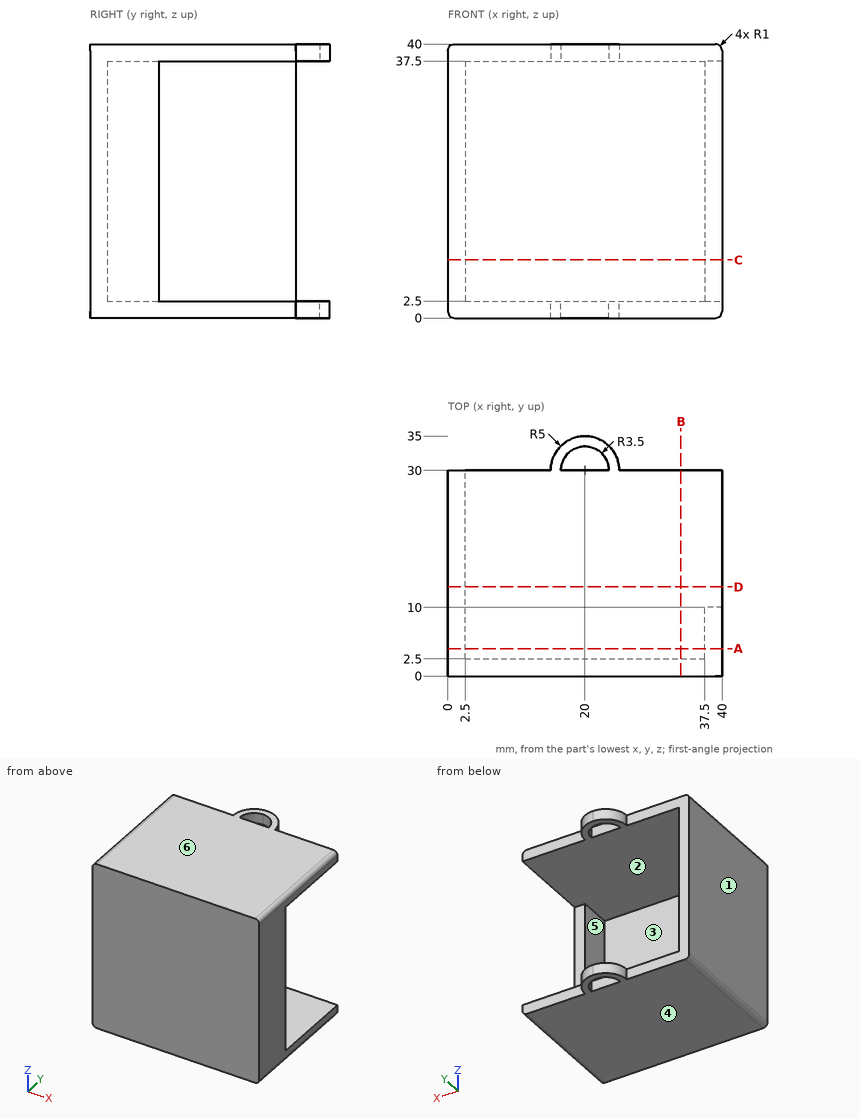
Check sheet for the drawn part. Datum: minimum x, y, z corner. Units: mm. A direction names the side the tool comes from. Give positions to 0.01 mm unless a question says otherwise; leave off trailing zeros. Write each loop counter-clockwise with the first axis right and the second up, starting at its lowest first coordinate (ties: lowest second). Pieces come first, ordered by that corner, then holes. Notation, with made-up numbers: (62.5, -34) - (113.5, -34) arc R25 cw to (113.5, 5) - close; hole circle Ø2 at (64, -39). An arc over 180 degrees is marked (long way). Put each result on its own line as item: value.
1. Sectioned sample at D-D, the plane y = 13. Enter the section's corners in (x, z), plus the area to 3 significant figures.
Ans:
outline: (0, 1) arc R1 ccw to (1, 0) - (39, 0) arc R1 ccw to (40, 1) - (40, 2.5) - (2.5, 2.5) - (2.5, 37.5) - (40, 37.5) - (40, 39) arc R1 ccw to (39, 40) - (1, 40) arc R1 ccw to (0, 39) - close
area: 287 mm²
2. Go/stop test with flat-tipped pins: pin 1 (0.8 mm diameter, centred on x = 38.5, z = 26, fed in from +Y); pin 2 (2 mm diameter, centred on x = 31, z = 38, fed in from +Y); pin 3 (1 mm diameter, centred on y = 19.5, z = 30.5, fed in from +X). Record where each tip stops, or that it passes through.
Ans:
pin 1: stops at y = 10
pin 2: stops at y = 30
pin 3: stops at x = 2.5
3. Sectioned sample at B-B, the plane x = 34. Enter the section's corners in (y, z).
Ans:
outline: (0, 0) - (30, 0) - (30, 2.5) - (2.5, 2.5) - (2.5, 37.5) - (30, 37.5) - (30, 40) - (0, 40) - close
4. Thickness scan on line 1 (Z direction, x = 36, y = 24); line 2 (Y direction, x = 29.5, z = 25). Record the ranges inside material, lowest first.
Ans:
line 1: z = 0 to 2.5, 37.5 to 40
line 2: y = 0 to 2.5
5. Sectioned sample at C-C, the plane z = 8.5. Enter the section's corners in (x, y), plus the area to 4 significant figures.
Ans:
outline: (0, 0) - (40, 0) - (40, 10) - (37.5, 10) - (37.5, 2.5) - (2.5, 2.5) - (2.5, 30) - (0, 30) - close
area: 187.5 mm²
6. Draft check along X on the marked faces 1, 2, 3 and 4. Enter one of: +X half, -X half, draft (parallel to the pull), parting line (faces both ways), or undercut.
Ans:
face 1: -X half
face 2: undercut
face 3: undercut
face 4: draft
7. Set-up check for the marked faces 5 and 6: record each of +Z, -Z, +X, -X, +Y, -Y from which the full face is reachable in a straight line by a thin tool's end or side.
Ans:
face 5: +Y
face 6: +Z, +X, -X, +Y, -Y
8. Sectioned sample at A-A, the plane y = 4. Enter the section's corners in (x, z), plus the area to 3 significant figures.
Ans:
outline: (0, 1) arc R1 ccw to (1, 0) - (39, 0) arc R1 ccw to (40, 1) - (40, 39) arc R1 ccw to (39, 40) - (1, 40) arc R1 ccw to (0, 39) - close; hole (2.5, 2.5) - (37.5, 2.5) - (37.5, 37.5) - (2.5, 37.5) - close
area: 374 mm²
